Autodesk Inventor part; units mm, degrees
ref_plane "YZ Plane" through (0, 0, 0) normal (1, 0, 0) x (0, 1, 0)
ref_plane "XZ Plane" through (0, 0, 0) normal (0, 1, 0) x (-1, 0, 0)
ref_plane "XY Plane" through (0, 0, 0) normal (0, 0, 1) x (1, 0, 0)
sketch "Sketch1" plane through (0, 0, 0) normal (0, 1, 0) x (-1, 0, 0)
  circle A0 centre (0, 0) radius 22.606
  circle A1 centre (0, 0) radius 16.002
  dimension "d4" = 32.004
  dimension "d5" = 45.212
extrude "Extrusion1" add sketch "Sketch1" against normal blind 127
sketch "Sketch2" plane through (0, 0, 0) normal (1, 0, 0) x (0, 1, 0)
  line L0 (0, 22.606) -> (-127, 22.606)
  circle A0 centre (0, 22.606) radius 3.175
  line L1 (0, 22.606) -> (0, -22.606) construction
  point P0 (0, 0)
  dimension "d18" = 6.35
  dimension "d23" = 0
coil "Coil1" sketch "Sketch2" operation cut axis through (0, -10, 0) along (0, -1, 0) pitch 50.8 turns 2.5 hand left
sketch "Sketch13" plane through (0, -127, 0) normal (0, -1, 0) x (1, 0, 0)
  circle A0 centre (0, 0) radius 25.146 construction
  arc A1 (8.6509, -20.8852) -> (0, -22.606) centre (0, 0) ccw construction
  line L0 (-1.3947, -15.9411) -> (-2.1121, -25.0571)
  line L1 (1.3947, -15.9411) -> (2.1121, -25.0571)
  line L2 (0, 0) -> (0, -25.146) construction
  circle A2 centre (0, 0) radius 16.002 construction
  arc A3 (-1.3947, -15.9411) -> (1.3947, -15.9411) centre (0, 0) ccw
  arc A4 (-2.1121, -25.0571) -> (2.1121, -25.0571) centre (0, 0) ccw
  dimension "d48" = 2.54
  dimension "d49" = 4.5
  dimension "d50" = 4.5
extrude "Extrusion6" add sketch "Sketch13" against normal blind 50.8
sketch "Sketch10" plane through (0, -127, 0) normal (0, -1, 0) x (1, 0, 0)
  line L0 (0, 0) -> (0, -22.606) construction
  arc A0 (8.6509, -20.8852) -> (0, -22.606) centre (0, 0) ccw construction
  arc A1 (0, -15.875) -> (3.175, -15.5543) centre (0, 0) ccw
  line L1 (3.175, -15.5543) -> (3.175, -25.781)
  line L2 (3.175, -25.781) -> (0, -25.781)
  arc A2 (-3.175, -15.5543) -> (0, -15.875) centre (0, 0) ccw
  line L3 (-3.175, -15.5543) -> (-3.175, -25.781)
  line L4 (-3.175, -25.781) -> (0, -25.781)
  dimension "d37" = 3.175
  dimension "d38" = 31.75
  dimension "d40" = 3.175
equation "\"d49\" = 0.5 * angleForSlot"
equation "\"d50\" = 0.5 * angleForSlot"
equation "\"angleForSlot\" = 9deg"
properties part number "InnerThreadedFocusTube" material "PBT Plastic"
Geometry: final body of the model. Coordinates: model frame, mm. A direction names the side the tool comes from. Give positions to 0.01 mm unless a question says otherwise; leave off trailing zeros. Put each result on its own line as item: value.
1. Pin query (flat end, axial travel): P1, Ø8, axis at y = -38.5, z = 16.5, coming from the +X side; P2, Ø1, axis at x = 11, y = -77, coming from the -Z side; P3, Ø6, axis at x = -11, y = -60, coming from the -Z side. Return the tip coordinate at first contact, or that it passes through.
Taken from the geometry:
P1: stops at x = 18.84
P2: stops at z = -20.02
P3: stops at z = -21.14
2. Ray query, line 1 along X through (y, z) = (-75.5, 0); line 2 along Y through (x, z) = (15, -13). Return the intervals inside material, ascending. Write a range as [from, to].
Taken from the geometry:
line 1: x = [-22.61, -16], [16, 22.61]
line 2: y = [-127, -121.65], [-118.5, -70.85], [-67.7, -20.05], [-16.9, 0]
3. Pull-direction query (Z, two-part tool) for faces 3 (the flat face through (-1.984, -101.956, -23.432)), 4 (the cylindrical face through (-0.03, -101.956, -25.146)), 5 (the flat face through (0, -1, 21)); classes: released by +Z, released by -Z, zero draft, split by the parting line, or undercut.
Taken from the geometry:
face 3: undercut
face 4: released by -Z
face 5: zero draft
4. Set-up query: faces 1 (the flat face through (0, -76.2, -22)), 2 (the flat face through (-10, 0, -15)). Return all of +Z, -Z, +X, -X, +Y, -Y with unobstructed straight access to the full face (end or side cutting, diameter ignored); none if empty.
Taken from the geometry:
face 1: -Z
face 2: +Z, -Z, +X, -X, +Y
